For this review, take the finished solid that the model builds, in its own axes (mm). A direction names the side the tool comes from. Coordinates: 2 decimals unless noted, no trailing zeros. Order: outer loops, then holes, each group sorted by start corner. A loop starts at its lowest first (then second) coordinate and runs counter-clockwise, first axis right, second up. Notation, with made-up numbers: (86, 15.25) - (100, 15.25) arc R27 ccw to (100, 43.25) - close; hole circle Ø11 at (-8, -14.75). An arc over 180 degrees is marked (long way). One line per item, written item: value. Start each with the question number.
(1) Clearance check with a flat-ended pin moving along its axis: pin 1 (1.3 mm diameter, centred on x = -7, y = 5, fed in from +Z). State where the tip first meets the part, or that it passes through.
(2) Consider section C-C on y = 3.75. Write out the cut boundary in (x, z), then the cut area to 3 significant figures.
(3) For faces 5 (the flat face through (-9, 7, 12.9)), 6 (the flat face through (-9, 6.439, 7)), list the 3-axis set-ups (+Z, -Z, +X, -X, +Y, -Y) from which the entire face can be reached by the end or side of a thin tool; tool diameter is ignored.
(4) Consider section A-A on z = 11.75. Write out the cut boundary in (x, y).
(5) Mouldability with a two-part tool opening along X and no side actions: class faces 1 (the flat face through (-9, 8.229, 6)), 2 (the flat face through (-9, 2.019, 7)), 3 (the flat face through (-1.043, 4, 6)), 4 (the flat face through (-14.443, 4, 7)) as released by +X, released by -X, zero draft, split by the parting line, or undercut.
(6) To check wall thickness, follow line 1 along Y through (x, z) = (-12.5, 6.25); line 2 along X through (y, z) = (5.25, 10.75); line 3 along Z through (x, y) = (-8, 5.25). State the ranges of each line that lie inside material, in increasing order.
(7) Consider section B-B on x = -5. Write out the cut boundary in (y, z), then the cut area to 3 significant figures.
```python
from build123d import *

# Parameters (mm, degrees)
F0_W     = 12
F0_H     = 4.42
F1_DEPTH = 2
F0_W_2   = 14.8
F0_H_2   = 8
F2_DEPTH = 12.9


with BuildPart() as f1:
    # F0 (on Top) → F1 (new body)
    with BuildSketch(Plane.XY):
        with Locations((-8.442831, 4.229229)):
            Rectangle(F0_W, F0_H)
    extrude(amount=F1_DEPTH)

    # F0 (on Top) → F2 (join)
    with BuildSketch(Plane.XY):
        with Locations((-8.442831, 4.229229)):
            Rectangle(F0_W_2, F0_H_2)
        with Locations((-8.442831, 4.229229)):
            Rectangle(F0_W, F0_H, mode=Mode.SUBTRACT)
    extrude(amount=F2_DEPTH)


solid = f1.part
```
Geometry check:
1. pin 1: stops at z = 2
2. outline: (-15.84, 0) - (-1.04, 0) - (-1.04, 12.9) - (-2.44, 12.9) - (-2.44, 2) - (-14.44, 2) - (-14.44, 12.9) - (-15.84, 12.9) - close
2. area: 60.1 mm^2
3. face 5: +Z, +X, -X, +Y, -Y
3. face 6: +Z
4. outline: (-15.84, 0.23) - (-1.04, 0.23) - (-1.04, 8.23) - (-15.84, 8.23) - close; hole (-14.44, 2.02) - (-2.44, 2.02) - (-2.44, 6.44) - (-14.44, 6.44) - close
5. face 1: zero draft
5. face 2: undercut
5. face 3: released by +X
5. face 4: undercut
6. line 1: y = 0.23 to 2.02, 6.44 to 8.23
6. line 2: x = -15.84 to -14.44, -2.44 to -1.04
6. line 3: z = 0 to 2
7. outline: (0.23, 0) - (8.23, 0) - (8.23, 12.9) - (6.44, 12.9) - (6.44, 2) - (2.02, 2) - (2.02, 12.9) - (0.23, 12.9) - close
7. area: 55.0 mm^2
